For this review, take the finished solid that the model builds, in its own axes (mm). Face numbers are marked on the shaded views. A direction names the side the tool comes from. Give positions to 0.01 mm unless a question says otherwise; leave off trailing zeros. Loops run counter-clockwise (first coordinate to the right, second up) from the corner with the lowest first, then second, coordinate; pieces in that order, holes last.
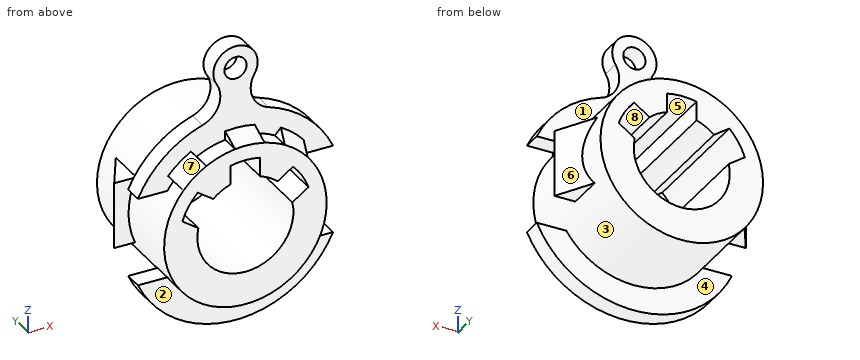
```python
from build123d import *

# Parameters (mm, degrees)
F0_R         = 44
F1_DEPTH     = 68
F3_R         = 6
F4_DEPTH     = 10
F7_DEPTH     = 10
F8_T4_ANGLE  = 83.7942350081
F8_T9_ANGLE  = 83.7884226617
F8_T14_ANGLE = 83.7665747307
F11_DEPTH    = 25
F12_T4_DEPTH = 165.3542877323
F12_S5_R     = 44
F12_T6_DEPTH = 86
F13_T4_DEPTH = 165.3542877323
F13_S5_R     = 44
F13_T6_DEPTH = 85


# Not quite as in the source:
# - a fillet or chamfer that OpenCascade refuses, or shapes differently, is made with other operations: its cross-section is extruded or revolved along the edge and cut away or added


with BuildPart() as f1:
    # F0 (on Front) → F1 (new body)
    with BuildSketch(Plane.XZ):
        Circle(F0_R)
        with BuildLine():
            ThreePointArc((-17.4170906965, 19.3040138746), (-12.9958030986, 22.5190830591), (-8, 24.7386337537))
            Line((-8, 24.7386337537), (-8, 35.0998575496))
            ThreePointArc((-8, 35.0998575496), (0, 36), (8, 35.0998575496))
            Line((8, 35.0998575496), (8, 24.7386337537))
            ThreePointArc((8, 24.7386337537), (12.9958030986, 22.5190830591), (17.4170906965, 19.3040138746))
            Line((17.4170906965, 19.3040138746), (25.7612918983, 25.1466864563))
            ThreePointArc((25.7612918983, 25.1466864563), (30.7135727536, 18.7796818053), (34.1239224392, 11.4698699802))
            Line((34.1239224392, 11.4698699802), (25.4359194285, 5.3864647801))
            ThreePointArc((25.4359194285, 5.3864647801), (0, -26), (-25.4359194285, 5.3864647801))
            Line((-25.4359194285, 5.3864647801), (-34.1239224392, 11.4698699802))
            ThreePointArc((-34.1239224392, 11.4698699802), (-30.7135727536, 18.7796818053), (-25.7612918983, 25.1466864563))
            Line((-25.7612918983, 25.1466864563), (-17.4170906965, 19.3040138746))
        make_face(mode=Mode.SUBTRACT)
    extrude(amount=F1_DEPTH)

    # F3 (on offset) → F4 (join)
    with BuildSketch(Plane.XZ.offset(48)):
        with BuildLine():
            ThreePointArc((-10.252187236, 75.7636022514), (-9.0876412514, 63.6171726174), (-17.8938638331, 55.1707317073))
            ThreePointArc((-17.8938638331, 55.1707317073), (-38.6311115614, 43.2624227191), (-52.8015151298, 24))
            Line((-52.8015151298, 24), (-36.8781778292, 24))
            ThreePointArc((-36.8781778292, 24), (0, 44), (36.8781778292, 24))
            Line((36.8781778292, 24), (52.8015151298, 24))
            ThreePointArc((52.8015151298, 24), (38.6311115614, 43.2624227191), (17.8938638331, 55.1707317073))
            ThreePointArc((17.8938638331, 55.1707317073), (9.0876412514, 63.6171726174), (10.252187236, 75.7636022514))
            ThreePointArc((10.252187236, 75.7636022514), (0, 94), (-10.252187236, 75.7636022514))
        make_face()
        with Locations((0, 82)):
            Circle(F3_R, mode=Mode.SUBTRACT)
        with BuildLine():
            ThreePointArc((36.8781778292, -24), (0, -44), (-36.8781778292, -24))
            Line((-36.8781778292, -24), (-52.8015151298, -24))
            ThreePointArc((-52.8015151298, -24), (0, -58), (52.8015151298, -24))
            Line((52.8015151298, -24), (36.8781778292, -24))
        make_face()
    extrude(amount=F4_DEPTH)

    # F6 (on offset) → F7 (join)
    with BuildSketch(Plane.XZ.offset(58)):
        with BuildLine():
            Line((-36.7577330787, 32.4016829643), (-33.5029734135, 28.5228114402))
            ThreePointArc((-33.5029734135, 28.5228114402), (-27.7578301996, 34.1394619555), (-21.0871377876, 38.6177759578))
            Line((-21.0871377876, 38.6177759578), (-24.3586089556, 42.5165634753))
            ThreePointArc((-24.3586089556, 42.5165634753), (-30.9738521636, 37.9686776455), (-36.7577330787, 32.4016829643))
        make_face()
        with BuildLine():
            ThreePointArc((-5.5873169023, 43.6438070043), (2.4537097938, 43.9315297736), (10.4126830977, 42.7501582536))
            Line((10.4126830977, 42.7501582536), (10.4126830977, 47.8808524434))
            ThreePointArc((10.4126830977, 47.8808524434), (2.4455798994, 48.9389327525), (-5.5873169023, 48.6804056046))
            Line((-5.5873169023, 48.6804056046), (-5.5873169023, 43.6438070043))
        make_face()
        with BuildLine():
            Line((33.6836647587, 28.3091986539), (37.1178360984, 31.9885329982))
            ThreePointArc((37.1178360984, 31.9885329982), (31.3875014297, 37.6274468175), (24.8122261451, 42.2534428624))
            Line((24.8122261451, 42.2534428624), (21.306338137, 38.4972720487))
            ThreePointArc((21.306338137, 38.4972720487), (27.9629096213, 33.9716894709), (33.6836647587, 28.3091986539))
        make_face()
    extrude(amount=F7_DEPTH)

    # F8: chamfer of 5 x 10.7225346025 on 3 edges, made by hand


with BuildPart() as f8_tool2:
    # F8_s3 → F8_t4 (revolve)
    with BuildSketch(Plane(origin=(0, 0, 0), x_dir=(0, 1, 0), z_dir=(0.1438242317, 0, -0.989603249))):
        Polygon((-68, 44), (-57.2774653975, 49), (-68, 49), align=None)
    revolve(axis=Axis((0, -68, 0), (0, -1, 0)), revolution_arc=F8_T4_ANGLE)

    split(bisect_by=Plane.XZ.offset(58), keep=Keep.TOP)


with BuildPart() as f1_1:
    add(f1.part)

    # F8_t1: cut F8_tool2
    add(f8_tool2.part, mode=Mode.SUBTRACT)


with BuildPart() as f8_tool7:
    # F8_s8 → F8_t9 (revolve)
    with BuildSketch(Plane(origin=(0, 0, 0), x_dir=(0, 1, 0), z_dir=(0.7101236851, 0, -0.7040769502))):
        Polygon((-68, 44), (-57.2774653975, 49), (-68, 49), align=None)
    revolve(axis=Axis((0, -68, 0), (0, -1, 0)), revolution_arc=F8_T9_ANGLE)

    split(bisect_by=Plane.XZ.offset(58), keep=Keep.TOP)


with BuildPart() as f1_2:
    add(f1_1.part)

    # F8_t6: cut F8_tool7
    add(f8_tool7.part, mode=Mode.SUBTRACT)


with BuildPart() as f8_tool12:
    # F8_s13 → F8_t14 (revolve)
    with BuildSketch(Plane(origin=(0, 0, 0), x_dir=(0, 1, 0), z_dir=(0.9989090113, 0, -0.0466988996))):
        Polygon((-68, 44), (-57.2774653975, 49), (-68, 49), align=None)
    revolve(axis=Axis((0, -68, 0), (0, -1, 0)), revolution_arc=F8_T14_ANGLE)

    split(bisect_by=Plane.XZ.offset(58), keep=Keep.TOP)


with BuildPart() as f1_3:
    add(f1_2.part)

    # F8_t11: cut F8_tool12
    add(f8_tool12.part, mode=Mode.SUBTRACT)

    # F10 (on offset) → F11 (join)
    with BuildSketch(Plane.XZ.offset(32)):
        with BuildLine():
            ThreePointArc((39.7816943244, 18.7993828803), (42.9324734337, 9.6334170917), (44, 0))
            ThreePointArc((44, 0), (43.1157719293, -8.7766856466), (40.4986267755, -17.2006171197))
            Line((40.4986267755, -17.2006171197), (51.7816943244, -17.2006171197))
            Line((51.7816943244, -17.2006171197), (51.7816943244, 18.7993828803))
            Line((51.7816943244, 18.7993828803), (39.7816943244, 18.7993828803))
        make_face()
        with BuildLine():
            ThreePointArc((-40.4986267755, -17.2006171197), (-43.9912774192, 0.8760770652), (-39.7816943244, 18.7993828803))
            Line((-39.7816943244, 18.7993828803), (-51.7816943244, 18.7993828803))
            Line((-51.7816943244, 18.7993828803), (-51.7816943244, -17.2006171197))
            Line((-51.7816943244, -17.2006171197), (-40.4986267755, -17.2006171197))
        make_face()
    extrude(amount=-F11_DEPTH)

    # F12: chamfer of 25 x 14.4337567297 on 1 edges, made by hand


with BuildPart() as f12_tool2:
    # F12_s3 → F12_t4 (new body)
    with BuildSketch(Plane.XY.offset(-81.8777609858)):
        with BuildLine():
            Line((36.8479375946, -6.1339745962), (52.2816943244, -32.8660254038))
            Line((52.2816943244, -32.8660254038), (52.7816943244, -32.8660254038))
            ThreePointArc((52.7816943244, -32.8660254038), (52.2816943244, -19.9330127019), (52.2816943244, -7))
            Line((52.2816943244, -7), (51.7816943244, -6.5))
            ThreePointArc((51.7816943244, -6.5), (44.3148159595, -6.5), (36.8479375946, -5.6339745962))
            Line((36.8479375946, -5.6339745962), (36.8479375946, -6.1339745962))
        make_face()
    extrude(amount=F12_T4_DEPTH)

    # F12_s5 → F12_t6 (cut, symmetric)
    with BuildSketch(Plane.XZ.offset(19.3)):
        Circle(F12_S5_R)
    extrude(amount=F12_T6_DEPTH, both=True, mode=Mode.SUBTRACT)


with BuildPart() as f1_4:
    add(f1_3.part)

    # F12_t1: cut F12_tool2
    add(f12_tool2.part, mode=Mode.SUBTRACT)

    # F13: chamfer of 25 x 14.4337567297 on 1 edges, made by hand


with BuildPart() as f13_tool2:
    # F13_s3 → F13_t4 (new body)
    with BuildSketch(Plane.XY.offset(83.4765267465)):
        Polygon((-37.3479375946, -7), (-51.7816943244, -32), (-51.7816943244, -7), align=None)
    extrude(amount=-F13_T4_DEPTH)

    # F13_s5 → F13_t6 (cut, symmetric)
    with BuildSketch(Plane.XZ.offset(19.5)):
        Circle(F13_S5_R)
    extrude(amount=F13_T6_DEPTH, both=True, mode=Mode.SUBTRACT)


with BuildPart() as f1_5:
    add(f1_4.part)

    # F13_t1: cut F13_tool2
    add(f13_tool2.part, mode=Mode.SUBTRACT)


solid = f1_5.part
```
Q1. Consider section C-C on y = -46. Give the boundary of the cut face in (x, z).
Answers:
outline: circle Ø88 at (0, 0); hole (-34.12, 11.47) - (-25.44, 5.39) arc R26 ccw (long way) to (25.44, 5.39) - (34.12, 11.47) arc R36 ccw to (25.76, 25.15) - (17.42, 19.3) arc R26 ccw to (8, 24.74) - (8, 35.1) arc R36 ccw to (-8, 35.1) - (-8, 24.74) arc R26 ccw to (-17.42, 19.3) - (-25.76, 25.15) arc R36 ccw to start
Q2. For probe 1 along Z at (x, y) = (0, -28); probe 2 along X at (y, z) = (-47, 0); probe 3 along Y at (x, z) = (-37, 30), list the stretches that pass through material, from the lowest coordinate up.
Answers:
probe 1: z = -44 to -26, 36 to 44
probe 2: x = -44 to -26, 26 to 44
probe 3: y = -58 to -48
Q3. Consider section D-D on z = 0. Give the boundary of the cut face in (x, y).
Answers:
outline: (-51.78, -32) - (-44, -32) - (-44, -68) - (-26, -68) - (-26, 0) - (-44, 0) - (-44, -18.52) - close; (26, -68) - (44, -68) - (44, -32) - (51.78, -32) - (44, -18.52) - (44, 0) - (26, 0) - close
Q4. Mouldability with a two-part tool opening along Z and no side actions: class the marked faces 6, 7 and 8 as +Z half, -Z half, draft (parallel to the pull), parting line (faces both ways), or undercut.
Answers:
face 6: draft
face 7: +Z half
face 8: undercut
Q5. Consider section A-A on x = 0. Give the boundary of the cut face in (y, z), plus the area to 3 significant figures.
Answers:
outline: (-68, -44) - (-58, -44) - (-58, -58) - (-48, -58) - (-48, -44) - (0, -44) - (0, -26) - (-68, -26) - close; (-68, 36) - (0, 36) - (0, 44) - (-48, 44) - (-48, 76) - (-58, 76) - (-58, 48.66) - (-68, 44) - close; (-58, 88) - (-48, 88) - (-48, 94) - (-58, 94) - close
area: 2,310 mm2
Q6. Machinability: for the marked faces 1, 2, 3, 4 and 5, which of the approach directions +Z, -Z, +X, -X, +Y, -Y give a long, thin tool a straight path to every point of the face, cutting with its end or side? Answer none if there is none.
Answers:
face 1: +Z, +Y
face 2: -Z, -Y
face 3: none
face 4: -Z, +Y
face 5: +Y, -Y
Q7. Consider section B-B on z = 82. Give the boundary of the cut face in (x, y), plus the area to 3 significant figures.
Answers:
outline: (-12, -58) - (-6, -58) - (-6, -48) - (-12, -48) - close; (6, -58) - (12, -58) - (12, -48) - (6, -48) - close
area: 120 mm2
Q8. For pin 1 Ø13 at (x, y) = (-46, -18.5) entering from +Z; pin 2 Ø1.5 at (y, z) = (-12, 37) entering from -X; pin 3 Ø8 at (x, y) = (31, -22) entering from -Z; pin 4 Ø12 at (x, z) = (23.5, 6.5) entering from +Y, all flat-tipped, find the tip position at first contact; note any pin that passes through.
Answers:
pin 1: stops at z = 19.38
pin 2: stops at x = -24.94
pin 3: stops at z = -34.74
pin 4: stops at y = 0
